Verification items for the finished model (mm, model axes). A direction names the side the tool comes from. Give positions to 0.01 mm unless a question says otherwise; leave off trailing zeros. Write each loop counter-clockwise with the first axis right and the second up, starting at its lowest first coordinate (ties: lowest second). Pieces come first, ordered by that corner, then holes. Notation, with made-up numbers: M 72,81 L 114,81 A32 ccw 114,114 Z; hole C -0.5,60 d3. An arc over 180 degrees is marked long. Answer as a JSON object with one key per item and string values.
Autodesk Inventor part; units mm, degrees
ref_plane "YZ Plane" through (0, 0, 0) normal (1, 0, 0) x (0, 1, 0)
ref_plane "XZ Plane" through (0, 0, 0) normal (0, 1, 0) x (-1, 0, 0)
ref_plane "XY Plane" through (0, 0, 0) normal (0, 0, 1) x (1, 0, 0)
sketch "Boceto1" plane through (0, 0, 0) normal (0, 1, 0) x (-1, 0, 0)
  circle A0 centre (0, 0) radius 16.5
  dimension "d0" = 33
extrude "Extrusión1" add sketch "Boceto1" along normal blind 30
sketch "Boceto2" plane through (0, 0, 0) normal (0, -1, 0) x (1, 0, 0)
  line L0 (-7.2902, 17.6) -> (7.2902, 17.6)
  line L1 (17.6, 7.2902) -> (17.6, -7.2902)
  line L2 (7.2902, -17.6) -> (-7.2902, -17.6)
  line L3 (-17.6, -7.2902) -> (-17.6, 7.2902)
  line L4 (-17.6, 17.6) -> (17.6, -17.6) construction
  line L5 (17.6, 17.6) -> (-17.6, -17.6) construction
  line L6 (-17.6, 7.2902) -> (-7.2902, 17.6)
  line L7 (-24.8902, 0) -> (10.3098, 0) construction
  line L8 (7.2902, 17.6) -> (17.6, 7.2902)
  line L9 (17.6, -7.2902) -> (7.2902, -17.6)
  line L10 (-7.2902, -17.6) -> (-17.6, -7.2902)
  line L11 (-24.8902, 0) -> (24.8902, 0)
  line L12 (0, -24.8902) -> (0, 24.8902)
  point P0 (0, 0)
  point P1 (0, 0)
  dimension "d3" = 35.2
  dimension "d4" = 35.2
  dimension "d5" = 35.2
  dimension "d6" = 45
  dimension "d7" = 35.2
extrude "Extrusión2" add sketch "Boceto2" against normal blind 4.9
fillet "Empalme1" radius 5 1 edges at (16.5, 30, 0)
sketch "Boceto3" plane through (0, 0, 0) normal (0, -1, 0) x (1, 0, 0)
  circle A0 centre (0, 0) radius 13.325
  dimension "d11" = 26.65
extrude "Extrusión3" cut sketch "Boceto3" against normal blind 25
properties part number "Tapón" material "PVC, no plastificado"
1) Section check A-A on y = 4. Record the boundary of the cut face in (x, z) (3 decimals), and give its area (3 significant figures).
Completed:
{"outline": "M -17.6,-7.29 L -7.29,-17.6 L 7.29,-17.6 L 17.6,-7.29 L 17.6,7.29 L 7.29,17.6 L -7.29,17.6 L -17.6,7.29 Z; hole C 0,0 d26.65", "area": "469 mm2"}
2) Section check D-D on y = 11.5. Record the boundary of the cut face in (x, z) (3 decimals), and give its area (3 significant figures).
Completed:
{"outline": "C 0,0 d33; hole C 0,0 d26.65", "area": "297 mm2"}
3) Section check C-C on x = 0. Record the boundary of the cut face in (y, z) (3 decimals), and give its area (3 significant figures).
Completed:
{"outline": "M 0,-17.6 L 4.9,-17.6 L 4.9,-16.5 L 25,-16.5 A5 ccw 30,-11.5 L 30,11.5 A5 ccw 25,16.5 L 4.9,16.5 L 4.9,17.6 L 0,17.6 L 0,13.325 L 25,13.325 L 25,-13.325 L 0,-13.325 Z", "area": "324 mm2"}
4) Thickness scan on L1, parallel to X at y = 16.5, z = -0.5; L2, parallel to Z at x = 0, y = 16.5 (3 decimals); L3, parallel to X at y = 2.5, z = -0.5. Record the ranges inside material, lowest first.
Completed:
{"L1": "x = -16.49 to -13.32, 13.32 to 16.49", "L2": "z = -16.5 to -13.325, 13.325 to 16.5", "L3": "x = -17.6 to -13.32, 13.32 to 17.6"}
5) Go/stop test with flat-tipped pins: pin 1 (5 mm diameter, centred on x = -8.5, z = 12.5, fed in from -Y); pin 2 (8 mm diameter, centred on x = 2, z = -2.5, fed in from -Y); pin 3 (12 mm diameter, centred on y = 15, z = 13.5, fed in from -X); pin 4 (6 mm diameter, centred on x = 2.5, y = 16, fed in from -Z). Record where each tip stops, or that it passes through.
Completed:
{"pin 1": "stops at y = 0", "pin 2": "stops at y = 25", "pin 3": "stops at x = -14.7", "pin 4": "stops at z = -16.5"}
6) Access from +Z, -Z, +X, -X, +Y, -Y to the whole of each face (thin tool, end or side, straight path). Record for faces 1 (the face through (-12.52, 2.42, 12.37)), 2 (the face through (9, 4.9, -14.3)).
Completed:
{"face 1": "+Z, -X, +Y, -Y", "face 2": "+Y"}
7) Section check B-B on z = 0. Record the boundary of the cut face in (x, y) (3 decimals).
Completed:
{"outline": "M -17.6,0 L -13.325,0 L -13.325,25 L 13.325,25 L 13.325,0 L 17.6,0 L 17.6,4.9 L 16.5,4.9 L 16.5,25 A5 ccw 11.5,30 L -11.5,30 A5 ccw -16.5,25 L -16.5,4.9 L -17.6,4.9 Z"}
8) Release check for a two-part mould opening along X. For faces 3 (the face through (-2.889, 12.325, -13.008)), 4 (the face through (-12.37, 2.42, -12.52)), 5 (the face through (12.37, 2.42, 12.52)), 6 (the face through (0, 25, 0)) record: pulls with the +X half, pulls with the -X half, needs draft (parallel to the pull), parting line crosses it, or undercut.
Completed:
{"face 3": "undercut", "face 4": "pulls with the -X half", "face 5": "pulls with the +X half", "face 6": "undercut"}
